Here's how the part is built. I have some questions about the finished solid (model axes, mm). Round coordinates to 2 decimals unless told otherwise and drop trailing zeros. Write each loop counter-clockwise with the first axis right and the second up, starting at its lowest first coordinate (ties: lowest second). Pieces come first, ordered by that corner, then holes. Notation, with made-up numbers: (77, 12) -> (83, 12) arc R19 ccw to (83, 39) -> close; hole circle Ø1 at (-22.5, -34). An arc over 180 degrees is marked (long way). Answer as CSV lines item,"result".
Solid Edge part; units mm, degrees
sketch "Sketch1" plane through (60.3162, 60.3162, 0) normal (0, 0, 1) x (1, 0, 0)
  line L0 (-110.3162, -97.8162) -> (-10.3162, -97.8162)
  line L1 (-10.3162, -97.8162) -> (-10.3162, -22.8162)
  line L2 (-10.3162, -22.8162) -> (-110.3162, -22.8162)
  line L3 (-110.3162, -22.8162) -> (-110.3162, -97.8162)
extrude "Protrusion1" add sketch "Sketch1" along normal blind 6
fillet "Verrundung_1" radius 5 1 edges at (50, 37.5, 3)
fillet "Verrundung_2" radius 5 3 edges at (50, -37.5, 3) (-50, -37.5, 3) (-50, 37.5, 3)
hole "Bohrung_1" at (0, 0, 6) direction (0, 0, -1) diameter 20 end up to next
hole "Bohrung_2" at (0, -30, 0) direction (0, 0, 1) diameter 4.5 end up to next countersink diameter 9 countersink angle 90
pattern_circular "Pattern1" count 4 over 360 about axis through (0, 0, 0) along (0, 0, 1) of "Bohrung_2"
hole "Bohrung_4" at (30, -30, 0) direction (0, 0, 1) diameter 3.242 end up to next thread major 4 thread length 10
hole "Hole1" at (30, 30, 0) direction (0, 0, 1) diameter 3.242 end up to next thread major 4 thread length 10
mirror "Mirror1" [suppressed]
properties material "Aluminium, 1060"
1. Suppose I cut it at B-B on x = -8. Please give me the cut outline in (y, z).
Numbers:
outline,"(-37.5, 0) -> (-6, 0) -> (-6, 6) -> (-37.5, 6) -> close; (6, 0) -> (37.5, 0) -> (37.5, 6) -> (6, 6) -> close"
2. For pin 1 Ø7 at (x, y) = (0, -30) entering from -Z, with a flat end and sliding along its axis, tell me the tip position at first contact or that it passes through.
Numbers:
pin 1,"stops at z = 1"
3. Suppose I cut it at A-A on y = -8. Please give me the cut outline in (x, z).
Numbers:
outline,"(-50, 0) -> (-6, 0) -> (-6, 6) -> (-50, 6) -> close; (6, 0) -> (50, 0) -> (50, 6) -> (6, 6) -> close"
4. If I drill on line 1 (Y direction, x = 0, z = 3.45); line 2 (Y direction, x = 30, z = 2.4); line 3 (X direction, y = 0, z = 4.7), over which ranges is the centre line in solid material (lowest first)?
Numbers:
line 1,"y = -37.5 to -32.25, -27.75 to -10, 10 to 27.75, 32.25 to 37.5"
line 2,"y = -37.5 to -31.62, -28.38 to -2.25, 2.25 to 28.38, 31.62 to 37.5"
line 3,"x = -50 to -32.25, -27.75 to -10, 10 to 27.75, 32.25 to 50"
5. If we mould it in two halves opening along Y, with no side actions, what happens to faces 1 (the face through (-12, 1, 0)), 2 (the face through (-9.76, 2.17, 3.04)), 3 (the face through (-48.5, 36.07, 3.04))? For each: released by +Y, released by -Y, zero draft, split by the parting line, or undercut.
Numbers:
face 1,"zero draft"
face 2,"undercut"
face 3,"released by +Y"
6. Suppose I cut it at C-C on y = -30. Please give me the cut outline in (x, z).
Numbers:
outline,"(-50, 0) -> (-4.5, 0) -> (-2.25, 2.25) -> (-2.25, 6) -> (-50, 6) -> close; (2.25, 2.25) -> (4.5, 0) -> (28.38, 0) -> (28.38, 6) -> (2.25, 6) -> close; (31.62, 0) -> (50, 0) -> (50, 6) -> (31.62, 6) -> close"
7. Suppose I cut it at D-D on x = 30. Please give me the cut outline in (y, z), and give its area (3 significant figures).
Numbers:
outline,"(-37.5, 0) -> (-31.62, 0) -> (-31.62, 6) -> (-37.5, 6) -> close; (-28.38, 0) -> (-4.5, 0) -> (-2.25, 2.25) -> (-2.25, 6) -> (-28.38, 6) -> close; (2.25, 2.25) -> (4.5, 0) -> (28.38, 0) -> (28.38, 6) -> (2.25, 6) -> close; (31.62, 0) -> (37.5, 0) -> (37.5, 6) -> (31.62, 6) -> close"
area,"379 mm^2"
